Read the model definition and answer for the solid it produces. Units are mm, in the model's axes. A direction names the side the tool comes from. Coordinates: 2 decimals unless noted, no trailing zeros. Order: outer loops, then holes, each group sorted by start corner. A loop starts at its lowest first (then second) coordinate and runs counter-clockwise, first axis right, second up. Notation, with made-up numbers: M -5.75,13 L 6.25,13 A12 ccw 6.25,29 Z; hole C 74.25,-24.75 d11. An arc over 180 degrees is marked long. Put each result on its own line as item: value.
from build123d import *

# Parameters (mm, degrees)
F0_W        = 508
F0_H        = 304.8
F1_DEPTH    = 50.8
F2_W        = 482.6
F2_H        = 273.05
F3_DEPTH    = 3.175
F4_R        = 2
F5_DEPTH    = 15
F6_W        = 88.9
F6_H        = 22.225
F7_DEPTH    = 25.4
F8_T1_DEPTH = 400.05
F8_T3_DEPTH = 495.3
F8_T5_DEPTH = 698.5
F8_T7_DEPTH = 400.05


# Not quite as in the source:
# - a fillet or chamfer that OpenCascade refuses, or shapes differently, is made with other operations: its cross-section is extruded or revolved along the edge and cut away or added


with BuildPart() as f1:
    # F0 (on Front) → F1 (new body)
    with BuildSketch(Plane.XZ):
        with Locations((0, 152.4)):
            Rectangle(F0_W, F0_H)
    extrude(amount=F1_DEPTH)

    # F2 (on face) → F3 (cut)
    with BuildSketch(Plane.XZ.offset(50.8)):
        with Locations((0, 155.575)):
            Rectangle(F2_W, F2_H)
    extrude(amount=-F3_DEPTH, mode=Mode.SUBTRACT)

    # F4 (on face) → F5 (cut)
    with BuildSketch(Plane(origin=(0, 0, 0), x_dir=(-1, 0, 0), z_dir=(0, 1, 0))):
        with Locations((-50, 207.95)):
            Circle(F4_R)
        with Locations((50, 207.95)):
            Circle(F4_R)
        with Locations((-50, 107.95)):
            Circle(F4_R)
        with Locations((50, 107.95)):
            Circle(F4_R)
    extrude(amount=-F5_DEPTH, mode=Mode.SUBTRACT)

    # F6 (on face) → F7 (cut)
    with BuildSketch(Plane(origin=(0, 0, 0), x_dir=(-1, 0, 0), z_dir=(0, 1, 0))):
        Polygon((177.8, 98.425), (-177.8, 98.425), (-177.8, 22.225), (-44.45, 22.225), (44.45, 22.225), (177.8, 22.225), align=None)
        with Locations((0, 11.1125)):
            Rectangle(F6_W, F6_H)
    extrude(amount=-F7_DEPTH, mode=Mode.SUBTRACT)

    # F8: fillet of radius 38.1 on 5 edges, made by hand

    # F8_s2 → F8_t1 (cut)
    with BuildSketch(Plane.YZ.offset(-50.8)):
        with BuildLine():
            ThreePointArc((-38.1, 0), (-11.1592316368, 11.1592316368), (0, 38.1))
            Line((0, 38.1), (0, 0))
            Line((0, 0), (-38.1, 0))
        make_face()
    extrude(amount=F8_T1_DEPTH, mode=Mode.SUBTRACT)

    # F8_s4 → F8_t3 (cut)
    with BuildSketch(Plane.XY.offset(-95.25)):
        with BuildLine():
            ThreePointArc((215.9, 0), (242.8407683632, -11.1592316368), (254, -38.1))
            Line((254, -38.1), (254, 0))
            Line((254, 0), (215.9, 0))
        make_face()
        with BuildLine():
            ThreePointArc((-254, -38.1), (-242.8407683632, -11.1592316368), (-215.9, 0))
            Line((-215.9, 0), (-254, 0))
            Line((-254, 0), (-254, -38.1))
        make_face()
    extrude(amount=F8_T3_DEPTH, mode=Mode.SUBTRACT)

    # F8_s6 → F8_t5 (cut)
    with BuildSketch(Plane.YZ.offset(-349.25)):
        with BuildLine():
            ThreePointArc((-38.1, 304.8), (-11.1592316368, 293.6407683632), (0, 266.7))
            Line((0, 266.7), (0, 304.8))
            Line((0, 304.8), (-38.1, 304.8))
        make_face()
    extrude(amount=F8_T5_DEPTH, mode=Mode.SUBTRACT)

    # F8_s8 → F8_t7 (cut)
    with BuildSketch(Plane.YZ.offset(-349.25)):
        with BuildLine():
            ThreePointArc((-38.1, 0), (-11.1592316368, 11.1592316368), (0, 38.1))
            Line((0, 38.1), (0, 0))
            Line((0, 0), (-38.1, 0))
        make_face()
    extrude(amount=F8_T7_DEPTH, mode=Mode.SUBTRACT)


solid = f1.part
Q1. Given pin 1 (6 mm diameter, centred on y = -18, z = 15.5, fed in from +X); pin 2 (22 mm diameter, centred on y = -17, z = 15, fed in from -X); pin 3 (6 mm diameter, centred on x = 39.5, z = 204.5, fed in from -Y) (3 decimals), each flat-ended and moving along its own axis, determine where each tip first touches the part or whether it passes through.
Answers below:
pin 1: stops at x = 249.95
pin 2: stops at x = -252.64
pin 3: stops at y = -47.625
Q2. A tool of negligible diameter and unlimited length cuts with its end or side. For faces 1 (the face through (112, -14, 22.225)), 2 (the face through (-254, -44, 150)), 3 (the face through (-3, -47.625, 157)), 4 (the face through (-44.45, -17, 14)), from which of +Z, -Z, +X, -X, +Y, -Y can it reach the whole face along a straight path? Write none if from no direction.
Answers below:
face 1: +Y
face 2: +Z, -Z, -X, +Y, -Y
face 3: -Y
face 4: -Z, +Y
Q3. Consider line 1 along X through (y, z) = (-4, 207); line 2 along X through (y, z) = (-9.5, 207.95); line 3 along Z through (x, y) = (50, -7) (3 decimals). Determine where each line is inside the solid, lowest interval first.
Answers below:
line 1: x = -232.89 to -51.76, -48.24 to 48.24, 51.76 to 232.89
line 2: x = -241.07 to -52, -48 to 48, 52 to 241.07
line 3: z = 16.091 to 22.225, 98.425 to 105.95, 109.95 to 205.95, 209.95 to 288.709
Q4. Find section B-B on z = 90. Write down the section's boundary in (x, y) (3 decimals).
Answers below:
outline: M -254,-50.8 L -241.3,-50.8 L -241.3,-47.625 L 241.3,-47.625 L 241.3,-50.8 L 254,-50.8 L 254,-38.1 A38.1 ccw 215.9,0 L 177.8,0 L 177.8,-25.4 L -177.8,-25.4 L -177.8,0 L -215.9,0 A38.1 ccw -254,-38.1 Z
Q5. Find section C-C on x = 145. Write down the section's boundary in (y, z) (3 decimals).
Answers below:
outline: M -50.8,0 L -38.1,0 A38.1 ccw -3.465,22.225 L -25.4,22.225 L -25.4,98.425 L 0,98.425 L 0,266.7 A38.1 ccw -38.1,304.8 L -50.8,304.8 L -50.8,292.1 L -47.625,292.1 L -47.625,19.05 L -50.8,19.05 Z
Q6. For a pull along Z with two mould halves and no side action, classify faces 5 (the face through (2, -25.4, 62)), 6 (the face through (-4, -44, 0)), 7 (the face through (-110, -14, 22.225)), 8 (the face through (254, -44, 150)) as +Z half, -Z half, draft (parallel to the pull), parting line (faces both ways), or undercut.
Answers below:
face 5: undercut
face 6: -Z half
face 7: undercut
face 8: draft
Q7. Find section A-A on x = 22.5. Write down the section's boundary in (y, z) (3 decimals), plus the area to 3 significant figures.
Answers below:
outline: M -50.8,0 L -38.1,0 A38.1 ccw -25.4,2.179 L -25.4,98.425 L 0,98.425 L 0,266.7 A38.1 ccw -38.1,304.8 L -50.8,304.8 L -50.8,292.1 L -47.625,292.1 L -47.625,19.05 L -50.8,19.05 Z
area: 11,800 mm^2
Q8. Find section D-D on z = 168.5. Write down the section's boundary in (x, y) (3 decimals).
Answers below:
outline: M -254,-50.8 L -241.3,-50.8 L -241.3,-47.625 L 241.3,-47.625 L 241.3,-50.8 L 254,-50.8 L 254,-38.1 A38.1 ccw 215.9,0 L -215.9,0 A38.1 ccw -254,-38.1 Z
